Source: CAD feature listing. Evaluate the final solid. Frame: model axes, mm. Face numbers are marked on the shaded views. Coordinates: 2 decimals unless noted, no trailing zeros. Order: outer loops, then holes, each group sorted by start corner. A loop starts at its lowest first (then second) coordinate and runs counter-clockwise, first axis right, second up.
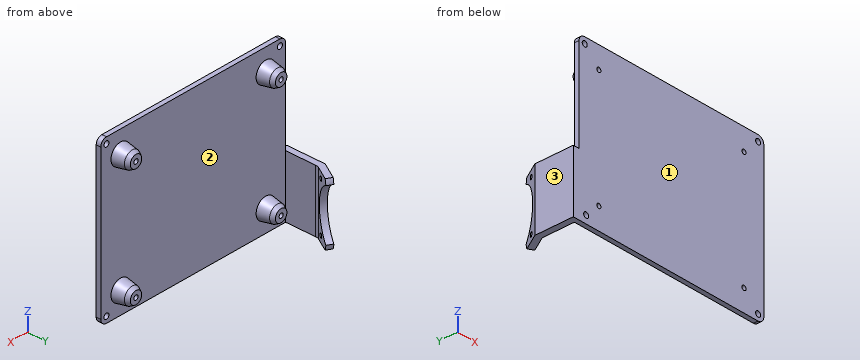
```python
from build123d import *
from OCP.BRepFilletAPI import BRepFilletAPI_MakeChamfer

# Parameters (mm, degrees)
SKETCH2_R                     = 1.75
BOSS_EXTRUDE1_DEPTH           = 3
BOSS_EXTRUDE2_START           = 10
SKETCH3_R                     = 5
BOSS_EXTRUDE2_DEPTH           = 13
BOSS_EXTRUDE2_DRAFT           = 10
BOSS_EXTRUDE2_PROFILE_2_DEPTH = 13
BOSS_EXTRUDE2_PROFILE_2_DRAFT = 10
BOSS_EXTRUDE2_PROFILE_3_DEPTH = 13
BOSS_EXTRUDE2_PROFILE_3_DRAFT = 10
BOSS_EXTRUDE2_PROFILE_4_DEPTH = 13
BOSS_EXTRUDE2_PROFILE_4_DRAFT = 10
SKETCH4_R                     = 1.45
CUT_EXTRUDE1_DEPTH            = 85.215198895
CHAMFER1_SIZE                 = 1
CHAMFER1_SIZE2                = 2.532088886
SKETCH5_W                     = 40
SKETCH5_H                     = 25
BOSS_EXTRUDE3_DEPTH           = 4
BOSS_EXTRUDE4_DEPTH           = 3
BOSS_EXTRUDE5_DEPTH           = 40
SKETCH8_R                     = 1.4
CUT_EXTRUDE3_DEPTH            = 4
FILLET1_R                     = 5


with BuildPart() as part:
    # Sketch2 → Boss-Extrude1 (new body)
    with BuildSketch(Plane(origin=(0, 0, 0), x_dir=(1, 0, 0), z_dir=(0, 1, 0))):
        with BuildLine():
            Line((-64.835, 47.15), (-64.835, -48.15))
            ThreePointArc((-64.835, -48.15), (-63.663427125, -50.978427125), (-60.835, -52.15))
            Line((-60.835, -52.15), (60.835, -52.15))
            ThreePointArc((60.835, -52.15), (63.663427125, -50.978427125), (64.835, -48.15))
            Line((64.835, -48.15), (64.835, 48.15))
            ThreePointArc((64.835, 48.15), (63.663427125, 50.978427125), (60.835, 52.15))
            Line((60.835, 52.15), (-59.835, 52.15))
            ThreePointArc((-59.835, 52.15), (-63.370533906, 50.685533906), (-64.835, 47.15))
        make_face()
        with Locations(Location((-59.835, 47.15, 0), (0, 0, 270))):
            Circle(SKETCH2_R, mode=Mode.SUBTRACT)
        with Locations(Location((60.835, 48.15, 0), (0, 0, 270))):
            Circle(SKETCH2_R, mode=Mode.SUBTRACT)
        with Locations(Location((60.835, -48.15, 0), (0, 0, 270))):
            Circle(SKETCH2_R, mode=Mode.SUBTRACT)
        with Locations(Location((-60.835, -48.15, 0), (0, 0, 270))):
            Circle(SKETCH2_R, mode=Mode.SUBTRACT)
    extrude(amount=BOSS_EXTRUDE1_DEPTH)


with BuildPart() as boss_extrude2_tool:
    # Sketch3 → Boss-Extrude2 (with draft: the straight prism first)
    with BuildSketch(Plane(origin=(0, 3, 0), x_dir=(1, 0, 0), z_dir=(0, 1, 0)).offset(BOSS_EXTRUDE2_START)):
        with Locations((-50.925, 38.05)):
            Circle(SKETCH3_R)
    extrude(amount=-BOSS_EXTRUDE2_DEPTH)
    # Boss-Extrude2: the draft: its side faces are tilted about the plane it starts from
    boss_extrude2_sides = [boss_extrude2_tool.faces().sort_by_distance(p)[0] for p in [
        (-55.925, 6.5, -38.05),
    ]]
    draft(boss_extrude2_sides, Plane(origin=(0, 3, 0), x_dir=(1, 0, 0), z_dir=(0, 1, 0)).offset(BOSS_EXTRUDE2_START), BOSS_EXTRUDE2_DRAFT)


with BuildPart() as part_1:
    add(part.part)

    # Boss-Extrude2: add boss_extrude2_tool
    add(boss_extrude2_tool.part)


with BuildPart() as boss_extrude2_profile_2_tool:
    # Sketch3 → Boss-Extrude2 profile 2 (with draft: the straight prism first)
    with BuildSketch(Plane(origin=(0, 3, 0), x_dir=(1, 0, 0), z_dir=(0, 1, 0)).offset(BOSS_EXTRUDE2_START)):
        with Locations((50.925, 38.05)):
            Circle(SKETCH3_R)
    extrude(amount=-BOSS_EXTRUDE2_PROFILE_2_DEPTH)
    # Boss-Extrude2 profile 2: the draft: its side faces are tilted about the plane it starts from
    boss_extrude2_profile_2_sides = [boss_extrude2_profile_2_tool.faces().sort_by_distance(p)[0] for p in [
        (45.925, 6.5, -38.05),
    ]]
    draft(boss_extrude2_profile_2_sides, Plane(origin=(0, 3, 0), x_dir=(1, 0, 0), z_dir=(0, 1, 0)).offset(BOSS_EXTRUDE2_START), BOSS_EXTRUDE2_PROFILE_2_DRAFT)


with BuildPart() as part_2:
    add(part_1.part)

    # Boss-Extrude2 profile 2: add boss_extrude2_profile_2_tool
    add(boss_extrude2_profile_2_tool.part)


with BuildPart() as boss_extrude2_profile_3_tool:
    # Sketch3 → Boss-Extrude2 profile 3 (with draft: the straight prism first)
    with BuildSketch(Plane(origin=(0, 3, 0), x_dir=(1, 0, 0), z_dir=(0, 1, 0)).offset(BOSS_EXTRUDE2_START)):
        with Locations((-50.925, -38.05)):
            Circle(SKETCH3_R)
    extrude(amount=-BOSS_EXTRUDE2_PROFILE_3_DEPTH)
    # Boss-Extrude2 profile 3: the draft: its side faces are tilted about the plane it starts from
    boss_extrude2_profile_3_sides = [boss_extrude2_profile_3_tool.faces().sort_by_distance(p)[0] for p in [
        (-55.925, 6.5, 38.05),
    ]]
    draft(boss_extrude2_profile_3_sides, Plane(origin=(0, 3, 0), x_dir=(1, 0, 0), z_dir=(0, 1, 0)).offset(BOSS_EXTRUDE2_START), BOSS_EXTRUDE2_PROFILE_3_DRAFT)


with BuildPart() as part_3:
    add(part_2.part)

    # Boss-Extrude2 profile 3: add boss_extrude2_profile_3_tool
    add(boss_extrude2_profile_3_tool.part)


with BuildPart() as boss_extrude2_profile_4_tool:
    # Sketch3 → Boss-Extrude2 profile 4 (with draft: the straight prism first)
    with BuildSketch(Plane(origin=(0, 3, 0), x_dir=(1, 0, 0), z_dir=(0, 1, 0)).offset(BOSS_EXTRUDE2_START)):
        with Locations((50.925, -38.05)):
            Circle(SKETCH3_R)
    extrude(amount=-BOSS_EXTRUDE2_PROFILE_4_DEPTH)
    # Boss-Extrude2 profile 4: the draft: its side faces are tilted about the plane it starts from
    boss_extrude2_profile_4_sides = [boss_extrude2_profile_4_tool.faces().sort_by_distance(p)[0] for p in [
        (45.925, 6.5, 38.05),
    ]]
    draft(boss_extrude2_profile_4_sides, Plane(origin=(0, 3, 0), x_dir=(1, 0, 0), z_dir=(0, 1, 0)).offset(BOSS_EXTRUDE2_START), BOSS_EXTRUDE2_PROFILE_4_DRAFT)


with BuildPart() as part_4:
    add(part_3.part)

    # Boss-Extrude2 profile 4: add boss_extrude2_profile_4_tool
    add(boss_extrude2_profile_4_tool.part)

    # Sketch4 → Cut-Extrude1 (cut, through all)
    with BuildSketch(Plane(origin=(0, 13, 0), x_dir=(1, 0, 0), z_dir=(0, 1, 0))):
        with Locations(Location((-50.925, 38.05, 0), (0, 0, 270))):
            Circle(SKETCH4_R)
        with Locations(Location((50.925, 38.05, 0), (0, 0, 270))):
            Circle(SKETCH4_R)
        with Locations(Location((50.925, -38.05, 0), (0, 0, 270))):
            Circle(SKETCH4_R)
        with Locations(Location((-50.925, -38.05, 0), (0, 0, 270))):
            Circle(SKETCH4_R)
    extrude(amount=-CUT_EXTRUDE1_DEPTH, mode=Mode.SUBTRACT)

    # Chamfer1: one chamfer whose edges measure the first distance from different faces: ONE call of the kernel's chamfer builder (chamfer() names one face for all edges)
    chamfer1_edges_1 = [part_4.edges().sort_by_distance(p)[0] for p in [
        (-55.925, 13, -38.05),
    ]]
    chamfer1_side_1 = [part_4.faces().sort_by_distance(p)[0] for p in [
        (-55.783578644, 13, -38.05),
    ]]
    chamfer1_edges_2 = [part_4.edges().sort_by_distance(p)[0] for p in [
        (45.925, 13, -38.05),
    ]]
    chamfer1_side_2 = [part_4.faces().sort_by_distance(p)[0] for p in [
        (46.066421356, 13, -38.05),
    ]]
    chamfer1_edges_3 = [part_4.edges().sort_by_distance(p)[0] for p in [
        (-55.925, 13, 38.05),
    ]]
    chamfer1_side_3 = [part_4.faces().sort_by_distance(p)[0] for p in [
        (-55.783578644, 13, 38.05),
    ]]
    chamfer1_edges_4 = [part_4.edges().sort_by_distance(p)[0] for p in [
        (45.925, 13, 38.05),
    ]]
    chamfer1_side_4 = [part_4.faces().sort_by_distance(p)[0] for p in [
        (46.066421356, 13, 38.05),
    ]]
    chamfer1 = BRepFilletAPI_MakeChamfer(part_4.part.solid().wrapped)
    for e in chamfer1_edges_1:
        chamfer1.Add(CHAMFER1_SIZE, CHAMFER1_SIZE2, e.wrapped, chamfer1_side_1[0].wrapped)  # the first distance lies on this face
    for e in chamfer1_edges_2:
        chamfer1.Add(CHAMFER1_SIZE, CHAMFER1_SIZE2, e.wrapped, chamfer1_side_2[0].wrapped)  # the first distance lies on this face
    for e in chamfer1_edges_3:
        chamfer1.Add(CHAMFER1_SIZE, CHAMFER1_SIZE2, e.wrapped, chamfer1_side_3[0].wrapped)  # the first distance lies on this face
    for e in chamfer1_edges_4:
        chamfer1.Add(CHAMFER1_SIZE, CHAMFER1_SIZE2, e.wrapped, chamfer1_side_4[0].wrapped)  # the first distance lies on this face
    add(Compound.cast(chamfer1.Shape()), mode=Mode.REPLACE)

    # Sketch5 → Boss-Extrude3 (add)
    with BuildSketch(Plane.ZY.offset(64.835)):
        with Locations((-32.15, 12.5)):
            Rectangle(SKETCH5_W, SKETCH5_H)
    extrude(amount=BOSS_EXTRUDE3_DEPTH)

    # Sketch6 → Boss-Extrude4 (add)
    with BuildSketch(Plane.XZ):
        with BuildLine():
            Line((-59.835, -52.15), (-64.835, -52.15))
            Line((-64.835, -52.15), (-64.835, -47.15))
            ThreePointArc((-64.835, -47.15), (-63.370533906, -50.685533906), (-59.835, -52.15))
        make_face()
    extrude(amount=-BOSS_EXTRUDE4_DEPTH)

    # Sketch7 → Boss-Extrude5 (add)
    with BuildSketch(Plane(origin=(0, 0, -52.15), x_dir=(-1, 0, 0), z_dir=(0, 0, -1))):
        Polygon((52.604700032, 45.111704166), (64.835, 23.92820323), (64.835, 25), (68.835, 25), (56.068801648, 47.111704166), align=None)
    extrude(amount=-BOSS_EXTRUDE5_DEPTH)

    # Sketch8 → Cut-Extrude3 (cut)
    with BuildSketch(Plane(origin=(-62.451567547, 36.056429335, 0), x_dir=(0, 0, 1), z_dir=(-0.866025403784438, 0.5000000000000011, 0))):
        with BuildLine():
            Line((-50.309630324, 12.765531799), (-52.15, 12.765531799))
            Line((-52.15, 12.765531799), (-52.15, 0.161338325))
            ThreePointArc((-52.15, 0.161338325), (-50.541368872, 0.867357709), (-48.817423041, 1.205245636))
            ThreePointArc((-48.817423041, 1.205245636), (-50.497778219, 6.864795081), (-50.309630324, 12.765531799))
        make_face()
        with BuildLine():
            Line((-13.990369676, 12.765531799), (-50.309630324, 12.765531799))
            ThreePointArc((-50.309630324, 12.765531799), (-50.497778219, 6.864795081), (-48.817423041, 1.205245636))
            ThreePointArc((-48.817423041, 1.205245636), (-32.15, -9.266864905), (-15.482576959, 1.205245636))
            ThreePointArc((-15.482576959, 1.205245636), (-14.1139621, 5.11593497), (-13.65, 9.233135095))
            ThreePointArc((-13.65, 9.233135095), (-13.735289019, 11.007513718), (-13.990369676, 12.765531799))
        make_face()
        with BuildLine():
            ThreePointArc((-13.990369676, 12.765531799), (-32.15, 27.733135095), (-50.309630324, 12.765531799))
            Line((-50.309630324, 12.765531799), (-13.990369676, 12.765531799))
        make_face()
        with BuildLine():
            Line((-12.15, 12.765531799), (-13.990369676, 12.765531799))
            ThreePointArc((-13.990369676, 12.765531799), (-13.735289019, 11.007513718), (-13.65, 9.233135095))
            ThreePointArc((-13.65, 9.233135095), (-14.1139621, 5.11593497), (-15.482576959, 1.205245636))
            ThreePointArc((-15.482576959, 1.205245636), (-13.758631128, 0.867357709), (-12.15, 0.161338325))
            Line((-12.15, 0.161338325), (-12.15, 12.765531799))
        make_face()
        with Locations(Location((-16.15, -6.766864905, 0), (0, 0, 270))):
            Circle(SKETCH8_R)
        with Locations(Location((-48.15, -6.766864905, 0), (0, 0, 270))):
            Circle(SKETCH8_R)
    extrude(amount=-CUT_EXTRUDE3_DEPTH, mode=Mode.SUBTRACT)

    # Fillet1
    fillet1_edges = [part_4.edges().sort_by_distance(p)[0] for p in [
        (-64.835, 23.92820323, -32.15),
    ]]
    fillet(fillet1_edges, radius=FILLET1_R)


solid = part_4.part
```
1. Section query A-A on z = 38.05. Return loops of the section in (x, y) (3 decimals), plus the area to 3 significant figures.
Findings:
outline: (-64.835, 0) - (-52.375, 0) - (-52.375, 13) - (-54.925, 13) - (-56.365, 10.506) - (-57.688, 3) - (-64.835, 3) - close; (-49.475, 0) - (49.475, 0) - (49.475, 13) - (46.925, 13) - (45.485, 10.506) - (44.162, 3) - (-44.162, 3) - (-45.485, 10.506) - (-46.925, 13) - (-49.475, 13) - close; (52.375, 0) - (64.835, 0) - (64.835, 3) - (57.688, 3) - (56.365, 10.506) - (54.925, 13) - (52.375, 13) - close
area: 544 mm2
2. Ray query, line 1 (X direction, y = 1.9, z = 48.15) (3 decimals); line 2 (X direction, y = 1, z = -48) (3 decimals); line 3 (X direction, y = 4.5, z = -38.05) (3 decimals). Return the intervals inside material, ascending.
Findings:
line 1: x = -64.835 to -62.585, -59.085 to 59.085, 62.585 to 64.835
line 2: x = -68.835 to -61.365, -58.305 to 59.091, 62.579 to 64.835
line 3: x = -68.835 to -64.835, -57.424 to -52.375, -49.475 to -44.426, 44.426 to 49.475, 52.375 to 57.424
3. Draft query along X for the marked faces 1, 2 and 3. Return one class per face: released by +X, released by -X, zero draft, split by the parting line, or undercut.
Findings:
face 1: zero draft
face 2: undercut
face 3: released by -X
4. Section query D-D on x = 37.5. Return loops of the section in (y, z), plus the area to 3 significant figures.
Findings:
outline: (0, -52.15) - (3, -52.15) - (3, 52.15) - (0, 52.15) - close
area: 313 mm2
5. Pin query (flat end, axial travel): P1, Ø9, axis at x = 51, z = 38.5, coming from the +Y side; P2, Ø5, axis at x = -64.5, y = 19, coming from the +Z side; P3, Ø12, axis at x = -28, z = -41, coming from the +Y side. Return the tip coordinate at first contact, or that it passes through.
Findings:
P1: stops at y = 13
P2: stops at z = -12.15
P3: stops at y = 3
6. Section query C-C on z = -26. Return loops of the section in (x, y) (3 decimals), plus the area to 3 significant figures.
Findings:
outline: (-68.835, 0) - (64.835, 0) - (64.835, 3) - (-64.835, 3) - (-64.835, 22.588) arc R5 cw to (-64.165, 25.088) - (-63.095, 26.942) - (-66.559, 28.942) - (-68.835, 25) - close
area: 503 mm2
7. Section query B-B on y = 7. Count the separate pieces of the cut face and the enclosed holes in it, plus the area to 3 significant figures.
Findings:
separate pieces: 5
enclosed holes: 4
area: 595 mm2
